```python
from build123d import *

# Parameters (mm, degrees)
F0_R      = 1.25
F1_DEPTH  = 2
F0_W      = 101
F0_H      = 73
F2_DEPTH  = 30
F3_DEPTH  = 33
F4_R      = 5.5
F5_DEPTH  = 2
F6_R      = 5.75
F7_DEPTH  = 2
F8_R      = 1
F9_R      = 5
F10_R     = 5
F10_R_2   = 1.8
F11_DEPTH = 5


# Not quite as in the source:
# - a feature names something its author has since deleted; it is built from what else it names


with BuildPart() as f1:
    # F0 (on Top) → F1 (new body)
    with BuildSketch(Plane.XY):
        with BuildLine():
            Line((41, -45), (49, -45))
            Line((49, -45), (49, -37))
            ThreePointArc((49, -37), (43.3431457505, -39.3431457505), (41, -45))
        make_face()
        with Locations((45.5, -41.5)):
            Circle(F0_R, mode=Mode.SUBTRACT)
        with BuildLine():
            Line((-41, -45), (41, -45))
            ThreePointArc((41, -45), (43.3431457505, -39.3431457505), (49, -37))
            Line((49, -37), (49, 17))
            ThreePointArc((49, 17), (43.3431457505, 19.3431457505), (41, 25))
            Line((41, 25), (-41, 25))
            ThreePointArc((-41, 25), (-43.3431457505, 19.3431457505), (-49, 17))
            Line((-49, 17), (-49, -37))
            ThreePointArc((-49, -37), (-43.3431457505, -39.3431457505), (-41, -45))
        make_face()
        with BuildLine():
            Line((-49, -45), (-41, -45))
            ThreePointArc((-41, -45), (-43.3431457505, -39.3431457505), (-49, -37))
            Line((-49, -37), (-49, -45))
        make_face()
        with Locations((-45.5, -41.5)):
            Circle(F0_R, mode=Mode.SUBTRACT)
        with BuildLine():
            Line((-49, 25), (-49, 17))
            ThreePointArc((-49, 17), (-43.3431457505, 19.3431457505), (-41, 25))
            Line((-41, 25), (-49, 25))
        make_face()
        with Locations((-45.5, 21.5)):
            Circle(F0_R, mode=Mode.SUBTRACT)
        with Locations((-45.5, 21.5)):
            Circle(F0_R)
        with BuildLine():
            ThreePointArc((41, 25), (43.3431457505, 19.3431457505), (49, 17))
            Line((49, 17), (49, 25))
            Line((49, 25), (41, 25))
        make_face()
        with Locations((45.5, 21.5)):
            Circle(F0_R, mode=Mode.SUBTRACT)
        with Locations((45.5, 21.5)):
            Circle(F0_R)
        with Locations((45.5, -41.5)):
            Circle(F0_R)
        with Locations((-45.5, -41.5)):
            Circle(F0_R)
    extrude(amount=F1_DEPTH)

    # F0 (on Top) → F2 (join)
    with BuildSketch(Plane.XY):
        with Locations((0, -10)):
            Rectangle(F0_W, F0_H)
        Polygon((49, -37), (49, -45), (41, -45), (-41, -45), (-49, -45), (-49, -37), (-49, 17), (-49, 25), (-41, 25), (41, 25), (49, 25), (49, 17), align=None, mode=Mode.SUBTRACT)
        with BuildLine():
            Line((-49, -45), (-41, -45))
            ThreePointArc((-41, -45), (-43.3431457505, -39.3431457505), (-49, -37))
            Line((-49, -37), (-49, -45))
        make_face()
        with Locations((-45.5, -41.5)):
            Circle(F0_R, mode=Mode.SUBTRACT)
        with BuildLine():
            Line((41, -45), (49, -45))
            Line((49, -45), (49, -37))
            ThreePointArc((49, -37), (43.3431457505, -39.3431457505), (41, -45))
        make_face()
        with Locations((45.5, -41.5)):
            Circle(F0_R, mode=Mode.SUBTRACT)
        with BuildLine():
            ThreePointArc((41, 25), (43.3431457505, 19.3431457505), (49, 17))
            Line((49, 17), (49, 25))
            Line((49, 25), (41, 25))
        make_face()
        with Locations((45.5, 21.5)):
            Circle(F0_R, mode=Mode.SUBTRACT)
        with BuildLine():
            Line((-49, 25), (-49, 17))
            ThreePointArc((-49, 17), (-43.3431457505, 19.3431457505), (-41, 25))
            Line((-41, 25), (-49, 25))
        make_face()
        with Locations((-45.5, 21.5)):
            Circle(F0_R, mode=Mode.SUBTRACT)
    extrude(amount=F2_DEPTH)

    # F0 (on Top) → F3 (join)
    with BuildSketch(Plane.XY):
        with Locations((0, -10)):
            Rectangle(F0_W, F0_H)
        Polygon((49, -37), (49, -45), (41, -45), (-41, -45), (-49, -45), (-49, -37), (-49, 17), (-49, 25), (-41, 25), (41, 25), (49, 25), (49, 17), align=None, mode=Mode.SUBTRACT)
    extrude(amount=F3_DEPTH)

    # F4 (on face) → F5 (cut)
    with BuildSketch(Plane.YZ.offset(50.5)):
        with Locations((0, 16)):
            Circle(F4_R)
    extrude(amount=-F5_DEPTH, mode=Mode.SUBTRACT)

    # F6 (on face) → F7 (cut)
    with BuildSketch(Plane.XZ.offset(46.5)):
        with Locations((-33, 16)):
            Circle(F6_R)
        with Locations((-11, 16)):
            Circle(F6_R)
        with Locations((11, 16)):
            Circle(F6_R)
        with Locations((33, 16)):
            Circle(F6_R)
    extrude(amount=-F7_DEPTH, mode=Mode.SUBTRACT)

    # F8
    f8_edges = [f1.edges().sort_by_distance(p)[0] for p in [
        (0, -45, 2),
        (-49, -10, 2),
        (0, 25, 2),
        (49, -10, 2),
        (43.343146, -39.343146, 2),
        (43.343146, 19.343146, 2),
        (-43.343146, 19.343146, 2),
        (-43.343146, -39.343146, 2),
    ]]
    fillet(f8_edges, radius=F8_R)

    # F9
    f9_edges = [f1.edges().sort_by_distance(p)[0] for p in [
        (-50.5, 26.5, 16.5),
        (50.5, 26.5, 16.5),
        (50.5, -46.5, 16.5),
        (-50.5, -46.5, 16.5),
        (49, -45, 31.5),
        (49, 25, 31.5),
        (-49, 25, 31.5),
        (-49, -45, 31.5),
    ]]
    fillet(f9_edges, radius=F9_R)

    # F10 (on face) → F11 (cut)
    with BuildSketch(Plane(origin=(0, 0, 0), x_dir=(1, 0, 0), z_dir=(0, 0, -1))):
        Circle(F10_R)
        with Locations((0, 9.5)):
            Circle(F10_R_2)
    extrude(amount=-F11_DEPTH, mode=Mode.SUBTRACT)


solid = f1.part
```
Input: part model. Units: mm. Frame: model coordinates. A direction names the side the tool comes from. Give positions to 0.01 mm unless a question says otherwise; leave off trailing zeros. Order: outer loops, then holes, each group sorted by start corner. A loop starts at its lowest first (then second) coordinate and runs counter-clockwise, first axis right, second up. Notation, with made-up numbers: M 57.25,-1 L 91.25,-1 A21 cw 91.25,25 Z; hole C 77,49.5 d3. An arc over 180 degrees is marked long. Return JSON: item names as keys, results as strings.
Item 1: First-contact query: P1, Ø4, axis at x = -44.5, y = 20, coming from the +Z side; P2, Ø10, axis at y = 0, z = 16, coming from the +X side; P3, Ø0.8, axis at x = 45.5, y = 22, coming from the +Z side. Flat tips, straight axial feed; report the tip coordinate or a pass-through.
Solutions:
{"P1": "z = 30", "P2": "x = -49", "P3": "z = 2"}
Item 2: Pull-direction query (Z, two-part tool) for faces 1 (the flat face through (-45, -40, 30)), 2 (the cylindrical face through (43.406, -39.281, 16.311)), 3 (the cylindrical face through (-27.688, -45.76, 13.798)); classes: +Z half, -Z half, draft (parallel to the pull), parting line (faces both ways), or undercut.
Solutions:
{"face 1": "+Z half", "face 2": "draft", "face 3": "undercut"}
Item 3: Cut plane D-D (z = 25). Return loops of the section in (x, y), then the cut area to 3 significant figures.
Solutions:
{"outline": "M -50.5,-41.5 A5 ccw -45.5,-46.5 L 45.5,-46.5 A5 ccw 50.5,-41.5 L 50.5,21.5 A5 ccw 45.5,26.5 L -45.5,26.5 A5 ccw -50.5,21.5 Z; hole M -49,-37 A8 cw -41,-45 L 41,-45 A8 cw 49,-37 L 49,17 A8 cw 41,25 L -41,25 A8 cw -49,17 Z; hole C -45.5,-41.5 d2.5; hole C -45.5,21.5 d2.5; hole C 45.5,-41.5 d2.5; hole C 45.5,21.5 d2.5", "area": "673 mm^2"}
Item 4: Cut plane A-A (y = -9.5). Return loops of the section in (x, z).
Solutions:
{"outline": "M -50.5,0 L -1.8,0 L -1.8,2 L -48,2 A1 cw -49,3 L -49,33 L -50.5,33 Z; M 1.8,0 L 50.5,0 L 50.5,33 L 49,33 L 49,3 A1 cw 48,2 L 1.8,2 Z"}
Item 5: Cut plane C-C (x = -11). Return loops of the section in (y, z).
Solutions:
{"outline": "M -46.5,0 L 26.5,0 L 26.5,33 L 25,33 L 25,3 A1 cw 24,2 L -44,2 A1 cw -45,3 L -45,10.25 L -46.5,10.25 Z; M -46.5,21.75 L -45,21.75 L -45,33 L -46.5,33 Z"}
Item 6: Ray query, probe 1 along Y at (x, z) = (24, 25); probe 2 along X at (y, z) = (21, 10.5); probe 3 along X at (y, z) = (-21, 23.5). Return the intervals inside material, ascending.
Solutions:
{"probe 1": "-46.5 to -45, 25 to 26.5", "probe 2": "-50.5 to -46.65, -44.35 to -42.07, 42.07 to 44.35, 46.65 to 50.5", "probe 3": "-50.5 to -49, 49 to 50.5"}
Item 7: Cut plane B-B (x = 0). Return loops of the section in (y, z), then the cut area to 3 significant figures.
Solutions:
{"outline": "M -46.5,0 L -11.3,0 L -11.3,2 L -44,2 A1 cw -45,3 L -45,33 L -46.5,33 Z; M -7.7,0 L -5,0 L -5,2 L -7.7,2 Z; M 5,0 L 26.5,0 L 26.5,33 L 25,33 L 25,3 A1 cw 24,2 L 5,2 Z", "area": "212 mm^2"}
Item 8: Access query for faces 4 (the cylindrical face through (-5.688, -45.76, 13.798)), 5 (the cylindrical face through (-43.281, -39.406, 16.311)), 6 (the cylindrical face through (-0.39, -7.743, 0.986)). Directions: +Z, -Z, +X, -X, +Y, -Y. A direction counts if a zero-diameter tool reaches every point of the face in a straight line with its end or side. Return the directions, or none.
Solutions:
{"face 4": "-Y", "face 5": "+Z", "face 6": "+Z, -Z"}
